Read the model definition and answer for the solid it produces. Units are mm, in the model's axes. A direction names the side the tool comes from. Coordinates: 2 decimals unless noted, no trailing zeros. Order: outer loops, then holes, each group sorted by start corner. A loop starts at its lowest first (then second) coordinate and runs counter-clockwise, first axis right, second up. Notation, with made-up numbers: (9.25, 9) - (26.25, 9) arc R24 ccw to (26.25, 48) - close; hole circle Ø5 at (0.5, 32). An arc over 180 degrees is marked (long way). Use one line per item in the form item = value.
```python
from build123d import *

# Parameters (mm, degrees)
F0_W        = 47
F0_H        = 133
F1_DEPTH    = 25
F2_W        = 41
F2_H        = 23
F3_DEPTH    = 131
F4_R        = 2
F5_R        = 2
F6_T1_DEPTH = 28
F6_S5_W     = 2
F6_S5_H     = 2
F6_T6_DEPTH = 2
F7_DEPTH    = 1
F8_DEPTH    = 1
F9_DEPTH    = 0.5


# Not quite as in the source:
# - a fillet or chamfer that OpenCascade refuses, or shapes differently, is made with other operations: its cross-section is extruded or revolved along the edge and cut away or added


with BuildPart() as f1:
    # F0 (on Top) → F1 (new body)
    with BuildSketch(Plane.XY):
        with Locations((-1.0670694858, 16.9100829363)):
            Rectangle(F0_W, F0_H)
    extrude(amount=F1_DEPTH)

    # F2 (on face) → F3 (cut, through all)
    with BuildSketch(Plane.XZ.offset(49.5899170637)):
        with Locations((-1.0670694858, 13.5)):
            Rectangle(F2_W, F2_H)
    extrude(amount=-F3_DEPTH, mode=Mode.SUBTRACT)

    # F4
    f4_edges = [f1.edges().sort_by_distance(p)[0] for p in [
        (22.432931, 16.910083, 0),
        (-1.067069, 83.410083, 0),
    ]]
    fillet(f4_edges, radius=F4_R)

    # F5
    f5_edges = [f1.edges().sort_by_distance(p)[0] for p in [
        (-24.567069, 15.910083, 0),
    ]]
    fillet(f5_edges, radius=F5_R)

    # F6: fillet of radius 2 on 1 edges, made by hand

    # F6_s2 → F6_t1 (cut)
    with BuildSketch(Plane.XY.offset(2)):
        with BuildLine():
            ThreePointArc((20.4329305142, 83.4100829363), (21.8471440766, 82.8242964987), (22.4329305142, 81.4100829363))
            Line((22.4329305142, 81.4100829363), (22.4329305142, 83.4100829363))
            Line((22.4329305142, 83.4100829363), (20.4329305142, 83.4100829363))
        make_face()
    extrude(amount=F6_T1_DEPTH, mode=Mode.SUBTRACT)


with BuildPart() as f6_tool4:
    # F6_s5 → F6_t6 (new body)
    with BuildSketch(Plane.XZ.offset(-81.4100829363)):
        with Locations((21.4329305142, 1)):
            Rectangle(F6_S5_W, F6_S5_H)
    extrude(amount=-F6_T6_DEPTH)

    # F6_s7 → F6_t8 (revolve, cut)
    with BuildSketch(Plane(origin=(20.4329305142, 81.4100829363, 2), x_dir=(-0.7071067812, 0, 0.7071067812), z_dir=(-0.7071067812, 0, -0.7071067812))):
        with BuildLine():
            ThreePointArc((0, -2), (2, 0), (0, 2))
            Line((0, 2), (0, -2))
        make_face()
    revolve(axis=Axis((20.4329305142, 81.4100829363, 2), (0, 1, 0)), mode=Mode.SUBTRACT)


with BuildPart() as f1_1:
    add(f1.part)

    # F6_t3: cut F6_tool4
    add(f6_tool4.part, mode=Mode.SUBTRACT)

    # F7 (add): a face of the model
    f7_faces = [f1_1.faces().sort_by_distance(p)[0] for p in [
        (-21.5670694858, 15.9100829363, 13.5),
    ]]
    extrude(f7_faces, amount=F7_DEPTH)

    # F8 (add): a face of the model
    f8_faces = [f1_1.faces().sort_by_distance(p)[0] for p in [
        (19.4329305142, 15.9100829363, 13.5),
    ]]
    extrude(f8_faces, amount=F8_DEPTH)

    # F9 (add): a face of the model
    f9_faces = [f1_1.faces().sort_by_distance(p)[0] for p in [
        (-20.5670694858, 15.9100829363, 13.5),
    ]]
    extrude(f9_faces, amount=-F9_DEPTH)


solid = f1_1.part
```
(1) Section A-A, the plane z = 17.5 is taken. Write down the section's boundary in (x, y), then the cut area to 3 significant figures.
Answer list:
outline = (-24.57, -49.59) - (-20.57, -49.59) - (-20.57, 81.41) - (18.43, 81.41) - (18.43, -49.59) - (22.43, -49.59) - (22.43, 81.41) arc R2 ccw to (20.43, 83.41) - (-22.57, 83.41) arc R2 ccw to (-24.57, 81.41) - close
area = 1,140 mm2
(2) Section B-B, the plane x = -1 is taken. Write down the section's boundary in (y, z).
Answer list:
outline = (-49.59, 0) - (81.41, 0) arc R2 ccw to (83.41, 2) - (83.41, 25) - (81.41, 25) - (81.41, 2) - (-49.59, 2) - close
(3) Which of the six approach directions +Z, -Z, +X, -X, +Y, -Y give full straight-line access (tool end or side, diameter ignored) to faces 1 (the flat face through (-20.567, 15, 13)), 2 (the flat face through (-1, -49.59, 1))?
Answer list:
face_1 = +Z, -Y
face_2 = +Z, -Z, +X, -X, -Y
(4) Section C-C, the plane y = 23.5 is taken. Write down the section's boundary in (x, z).
Answer list:
outline = (-24.57, 2) arc R2 ccw to (-22.57, 0) - (20.43, 0) arc R2 ccw to (22.43, 2) - (22.43, 25) - (18.43, 25) - (18.43, 2) - (-20.57, 2) - (-20.57, 25) - (-24.57, 25) - close
(5) The mould has two halves that part along X. Classify faces 3 (the flat face through (-1, 81.41, 14)), 4 (the flat face through (22.433, 15, 13)), 5 (the flat face through (-24.567, 15, 13)), 6 (the flat face through (-1, 17, 0)): +X half, -X half, draft (parallel to the pull), parting line (faces both ways), or undercut.
Answer list:
face_3 = undercut
face_4 = +X half
face_5 = -X half
face_6 = draft
(6) Given pin 1 Ø8 at (x, z) = (-14.5, 10) entering from -Y; pin 2 Ø5 at (x, y) = (3.5, 14.5) entering from +Z, each flat-ended and moving along its own axis, determine where each tip first touches the part or whether it passes through.
Answer list:
pin_1 = 81.41
pin_2 = 2
(7) Straight lines are drawn through the part: L1, parallel to X at y = 4, z = 21.25; L2, parallel to Z at x = 14, y = 0.5; L3, parallel to Y at x = -11, z = 13.5. For each, find the intervals that lie inside material, in ascending order.
Answer list:
L1 = -24.57 to -20.57, 18.43 to 22.43
L2 = 0 to 2
L3 = 81.41 to 83.41
